Could you check a few things on this model? Use its own coordinates, in mm. Round coordinates to 2 decimals unless told otherwise and drop trailing zeros. Write each loop counter-clockwise with the first axis right and the second up, starting at its lowest first coordinate (ties: lowest second). Pieces come first, ordered by that corner, then holes. Notation, with made-up numbers: (21, 56.25) - (76, 56.25) arc R5 ccw to (76, 61.25) - close; hole circle Ø8 at (86, -6.5). An arc over 180 degrees is marked (long way). Write each question's results on one line, items separated by ' | '. Start each with the question number.
(1) Imagine slicing it at A-A on y = 0. Write out the boundary of the cut face in (x, z).
(2) Thinking about a two-plate mould opening in Y: for faces 1 (the flat face through (-1, 5, 0)), 2 (the cylindrical face through (3.78, 2.9, 25.35)), which applies, +Y half, -Y half, draft (parallel to the pull), parting line (faces both ways), or undercut?
(3) For P1, Ø1, axis at x = -3.5, z = 22, coming from the +Y side; P2, Ø2, axis at y = 4.5, z = 36, coming from the +X side; P3, Ø5, axis at y = 2.5, z = 43, coming from the +X side; P4, Ø1, axis at x = 1.5, z = 24.5, coming from the +Y side, each with a flat end and sliding along its axis, tell me the tip position at first contact or that it passes through.
(4) Please list where these lines run through material, in increasing order: line 1 (Y direction, x = 0, z = 36.5); line 2 (Y direction, x = -4, z = 26). Write a range as [from, to].
```python
from build123d import *

# Parameters (mm, degrees)
BOSS_EXTRUDE1_DEPTH        = 50
F_3_8_0_3750_DOWEL_HOLE1_D = 9.525


with BuildPart() as part:
    # Sketch1 → Boss-Extrude1 (new body)
    with BuildSketch(Plane.XY):
        with BuildLine():
            Line((6.148361062, 1.5875), (3.862361062, 1.5875))
            Line((3.862361062, 1.5875), (3.862361062, -1.5875))
            Line((3.862361062, -1.5875), (6.148361062, -1.5875))
            ThreePointArc((6.148361062, -1.5875), (-6.35, 0), (6.148361062, 1.5875))
        make_face()
        with BuildLine():
            ThreePointArc((6.148361062, 1.5875), (6.35, 0), (6.148361062, -1.5875))
            Line((6.148361062, -1.5875), (3.862361062, -1.5875))
            Line((3.862361062, -1.5875), (3.862361062, 1.5875))
            Line((3.862361062, 1.5875), (6.148361062, 1.5875))
        make_face()
    extrude(amount=BOSS_EXTRUDE1_DEPTH)

    # 3/8 (0.3750) Dowel Hole1 (through all)
    with Locations(Plane(origin=(0, 0, 0), x_dir=(1, 0, 0), z_dir=(0, 0, -1))):
        with Locations((0, 0)):
            Hole(F_3_8_0_3750_DOWEL_HOLE1_D / 2)

    # Sketch5 → Cut-Revolve1 (revolve, cut)
    with BuildSketch(Plane(origin=(0, 0, 0), x_dir=(1, 0, 0), z_dir=(0, 1, 0))):
        with BuildLine():
            ThreePointArc((-6.35, -44.05), (-5.9055, -44.4945), (-6.35, -44.939))
            Line((-6.35, -44.939), (-6.35, -44.05))
        make_face()
        with BuildLine():
            Line((-6.35, -5.95), (-6.35, -5.061))
            ThreePointArc((-6.35, -5.061), (-5.9055, -5.5055), (-6.35, -5.95))
        make_face()
    revolve(axis=Axis((0, 0, 50), (0, 0, -1)), mode=Mode.SUBTRACT)


solid = part.part
```
Response:
1) outline: (-6.35, 0) - (-4.76, 0) - (-4.76, 50) - (-6.35, 50) - (-6.35, 44.94) arc R0.44 cw to (-6.35, 44.05) - (-6.35, 5.95) arc R0.44 cw to (-6.35, 5.06) - close; (4.76, 0) - (6.35, 0) - (6.35, 5.06) arc R0.44 cw to (6.35, 5.95) - (6.35, 44.05) arc R0.44 cw to (6.35, 44.94) - (6.35, 50) - (4.76, 50) - close
2) face 1: draft | face 2: undercut
3) P1: y = 5.6 | P2: x = 5.3 | P3: x = 6.35 | P4: y = 6.27
4) line 1: [-6.35, -4.76], [4.76, 6.35] | line 2: [-4.93, -2.58], [2.58, 4.93]
